Source: CAD feature listing. Evaluate the final solid. Frame: model axes, mm. Face numbers are marked on the shaded views. Round coordinates to 2 decimals unless told otherwise and drop trailing zeros. Loops run counter-clockwise (first coordinate to the right, second up) from the corner with the lowest first, then second, coordinate; pieces in that order, holes last. Notation, with made-up numbers: M 27,50.5 L 56,50.5 A19 ccw 56,63.5 Z; hole C 88,-31.75 d6. An arc over 180 degrees is marked long. Write each question's results on one line, items separated by ' | '. Start each with the question number.
1. Contact query for flat-ended pins moving along their axis: pin 1 Ø1.5 at (x, z) = (10, 2.5) entering from +Y; pin 2 Ø0.9 at (y, z) = (-6, 6.5) entering from -X; pin 3 Ø3 at (x, z) = (16, 6.5) entering from -Y; pin 4 Ø5 at (x, y) = (1.5, -1.5) entering from +Z. Output: stop coordinate, or through.
2. Draft query along X for the marked faces 1 and 2. Return one class per face: released by +X, released by -X, zero draft, split by the parting line, or undercut.
3. Section B-B on z = 6.25. Output: boundary loops of the cut face in (x, y), and give its area (3 significant figures).
4. Section A-A on x = 0. Output: boundary loops of the cut face in (y, z).
5. Section C-C on x = 8.5. Output: boundary loops of the cut face in (y, z), and give its area (3 significant figures).
6. Ray query, line 1 (Y direction, x = 1, z = 2.25); line 2 (Y direction, x = 24.5, z = 3.25); line 3 (Y direction, x = 17, z = 8.25). Return the intervals inside material, ascending.
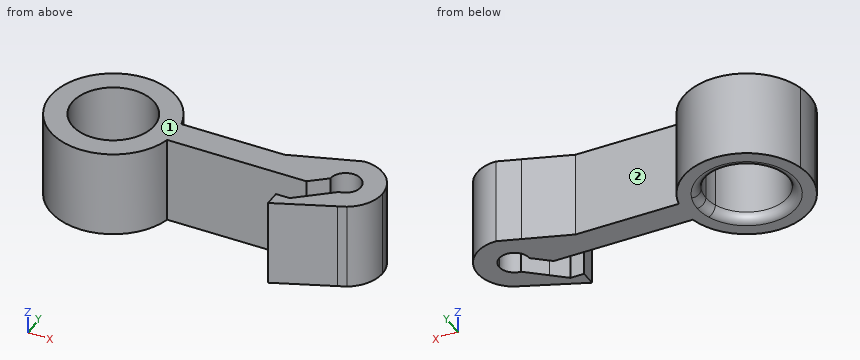
from build123d import *

# Parameters (mm, degrees)
F1_DEPTH = 10
F2_R     = 1


# Not quite as in the source:
# - a feature names something its author has since deleted; it is built from what else it names


with BuildPart() as f1:
    # F0 (on Top) → F1 (new body)
    with BuildSketch(Plane.XY):
        with BuildLine():
            ThreePointArc((-4.4255569592, 1.5825440281), (0, 4.7), (4.4255569592, 1.5825440281))
            Line((4.4255569592, 1.5825440281), (7.0239272775, 1.5825440281))
            ThreePointArc((7.0239272775, 1.5825440281), (0, 7.2), (-7.0239272775, 1.5825440281))
            Line((-7.0239272775, 1.5825440281), (-4.4255569592, 1.5825440281))
        make_face()
        with BuildLine():
            ThreePointArc((-4.4255569592, -1.5825440281), (-4.7, 0), (-4.4255569592, 1.5825440281))
            Line((-4.4255569592, 1.5825440281), (-7.0239272775, 1.5825440281))
            ThreePointArc((-7.0239272775, 1.5825440281), (-7.2, 0), (-7.0239272775, -1.5825440281))
            Line((-7.0239272775, -1.5825440281), (-4.4255569592, -1.5825440281))
        make_face()
        with BuildLine():
            Line((7.0239272775, -1.5825440281), (4.4255569592, -1.5825440281))
            ThreePointArc((4.4255569592, -1.5825440281), (0, -4.7), (-4.4255569592, -1.5825440281))
            Line((-4.4255569592, -1.5825440281), (-7.0239272775, -1.5825440281))
            ThreePointArc((-7.0239272775, -1.5825440281), (0, -7.2), (7.0239272775, -1.5825440281))
        make_face()
        with BuildLine():
            ThreePointArc((4.4255569592, 1.5825440281), (4.6308810019, 0.8030822784), (4.7, 0))
            ThreePointArc((4.7, 0), (4.6308810019, -0.8030822784), (4.4255569592, -1.5825440281))
            Line((4.4255569592, -1.5825440281), (7.0239272775, -1.5825440281))
            ThreePointArc((7.0239272775, -1.5825440281), (7.1558464348, -0.7961543827), (7.2, 0))
            ThreePointArc((7.2, 0), (7.1558464348, 0.7961543827), (7.0239272775, 1.5825440281))
            Line((7.0239272775, 1.5825440281), (4.4255569592, 1.5825440281))
        make_face()
        with BuildLine():
            ThreePointArc((24.1954502469, 3.3965829239), (23.3763263872, 2.5847294548), (22.8056300377, 1.5825440281))
            Line((22.8056300377, 1.5825440281), (25, 1.5825440281))
            Line((25, 1.5825440281), (25, 0))
            ThreePointArc((25, 0), (26.75, 1.75), (28.5, 0))
            ThreePointArc((28.5, 0), (28.0337651782, -1.1893052456), (26.8834891802, -1.7449013264))
            Line((26.8834891802, -1.7449013264), (24.5703446749, -3.6485069089))
            ThreePointArc((24.5703446749, -3.6485069089), (26.1897753497, -4.2129144711), (27.9004272408, -4.0913343989))
            Line((27.9004272408, -4.0913343989), (28.8181424703, -3.7128542555))
            ThreePointArc((28.8181424703, -3.7128542555), (30.41415785, -2.1532411037), (31, 0))
            ThreePointArc((31, 0), (29.7329020897, 3.0273412631), (26.6871552362, 4.2495353317))
            Line((26.6871552362, 4.2495353317), (24.1954502469, 3.3965829239))
        make_face()
        with BuildLine():
            ThreePointArc((22.8056300377, 1.5825440281), (22.5, 0), (22.8056300377, -1.5825440281))
            Line((22.8056300377, -1.5825440281), (23.0520843585, -1.5825440281))
            Line((23.0520843585, -1.5825440281), (25, 0))
            Line((25, 0), (25, 1.5825440281))
            Line((25, 1.5825440281), (22.8056300377, 1.5825440281))
        make_face()
        with BuildLine():
            Line((18.896151334, 1.5825440281), (7.0239272775, 1.5825440281))
            ThreePointArc((7.0239272775, 1.5825440281), (7.1558464348, 0.7961543827), (7.2, 0))
            ThreePointArc((7.2, 0), (7.1558464348, -0.7961543827), (7.0239272775, -1.5825440281))
            Line((7.0239272775, -1.5825440281), (22.8056300377, -1.5825440281))
            ThreePointArc((22.8056300377, -1.5825440281), (22.5, 0), (22.8056300377, 1.5825440281))
            Line((22.8056300377, 1.5825440281), (18.896151334, 1.5825440281))
        make_face()
        with BuildLine():
            Line((24.1954502469, 3.3965829239), (18.896151334, 1.5825440281))
            Line((18.896151334, 1.5825440281), (22.8056300377, 1.5825440281))
            ThreePointArc((22.8056300377, 1.5825440281), (23.3763263872, 2.5847294548), (24.1954502469, 3.3965829239))
        make_face()
        with BuildLine():
            ThreePointArc((27.9004272408, -4.0913343989), (26.1897753497, -4.2129144711), (24.5703446749, -3.6485069089))
            Line((24.5703446749, -3.6485069089), (22.897355554, -5.0252957012))
            Line((22.897355554, -5.0252957012), (21.3165715317, -5.0252957012))
            Line((21.3165715317, -5.0252957012), (21.3165715317, -6.8066196779))
            Line((21.3165715317, -6.8066196779), (27.9004272408, -4.0913343989))
        make_face()
    extrude(amount=F1_DEPTH)

    # F2
    f2_edges = [f1.edges().sort_by_distance(p)[0] for p in [
        (-4.425557, -1.582544, 0),
    ]]
    fillet(f2_edges, radius=F2_R)


solid = f1.part
Taken from the geometry:
1) pin 1: y = 1.58 | pin 2: x = -4.59 | pin 3: y = -1.58 | pin 4: through
2) face 1: zero draft | face 2: undercut
3) outline: M 7.02,-1.58 L 23.05,-1.58 L 25,0 A1.75 cw long 26.88,-1.74 L 22.9,-5.03 L 21.32,-5.03 L 21.32,-6.81 L 28.82,-3.71 A4.25 ccw 26.69,4.25 L 18.9,1.58 L 7.02,1.58 A7.2 ccw long Z; hole C 0,0 d9.4 | area: 193 mm^2
4) outline: M -7.2,0 L -5.7,0 A1 ccw -4.7,1 L -4.7,10 L -7.2,10 Z; M 4.7,1 A1 ccw 5.7,0 L 7.2,0 L 7.2,10 L 4.7,10 Z
5) outline: M -1.58,0 L 1.58,0 L 1.58,10 L -1.58,10 Z | area: 31.7 mm^2
6) line 1: -7.13 to -4.59, 4.59 to 7.13 | line 2: -5.49 to -3.71, -0.41 to 3.5 | line 3: -1.58 to 1.58
